from build123d import *

# Parameters (mm, degrees)
SKETCH_1_R               = 4
EXTRUDE_1_DEPTH          = 147.8
SKETCH_2_R               = 3
EXTRUDE_2_DEPTH          = 5
CUT_EXTRUDE_1_DEPTH      = 153.904676187
CUT_EXTRUDE_1_DEPTH_BACK = 153.904676187
SKETCH_3_R               = 1.65


with BuildPart() as part:
    # ｽｹｯﾁ1 → ﾎﾞｽ - 押し出し1 (new body)
    with BuildSketch(Plane.XY):
        Circle(SKETCH_1_R)
    extrude(amount=EXTRUDE_1_DEPTH)

    # ｽｹｯﾁ2 → ﾎﾞｽ - 押し出し2 (add)
    with BuildSketch(Plane.XY.offset(147.8)):
        Circle(SKETCH_2_R)
    extrude_2 = extrude(amount=EXTRUDE_2_DEPTH)

    # ﾐﾗｰ1: ﾎﾞｽ - 押し出し2 across plane
    add(extrude_2.mirror(Plane.XY.offset(73.9)))

    # ｽｹｯﾁ3 → ｶｯﾄ - 押し出し1 (cut, two sides: drawn at the far end of the back side and taken through both)
    with BuildSketch(Plane(origin=(0, 0, 0), x_dir=(1, 0, 0), z_dir=(0, 1, 0)).offset(-CUT_EXTRUDE_1_DEPTH_BACK)):
        with Locations(Location((0, -63.9, 0), (0, 0, 270))):
            Circle(SKETCH_3_R)
        with Locations(Location((0, -83.9, 0), (0, 0, 270))):
            Circle(SKETCH_3_R)
    extrude(amount=CUT_EXTRUDE_1_DEPTH + CUT_EXTRUDE_1_DEPTH_BACK, mode=Mode.SUBTRACT)


solid = part.part
Here's how the part is built. I have some questions about the finished solid (model axes, mm). A direction names the side the tool comes from. Round coordinates to 2 decimals unless told otherwise and drop trailing zeros. Order: outer loops, then holes, each group sorted by start corner. A loop starts at its lowest first (then second) coordinate and runs counter-clockwise, first axis right, second up. Notation, with made-up numbers: M -21.5,-34 L 11.5,-34 A13 ccw 11.5,-15 Z; hole C 10,76.5 d10. An arc over 180 degrees is marked long. Return JSON: item names as keys, results as strings. Group by question number.
1. On a 3-axis mill with a long thin cutter (end or side, diameter ignored), from which of +Z, -Z, +X, -X, +Y, -Y can I reach the whole of each face in a straight line? I mean faces 1 (the face through (1, 3, 0)), 2 (the face through (0, 0, -5)), 3 (the face through (-3, 0, 150)). Say none if no direction works.
2. Please list where these lines run through material, in increasing order: probe 1 along Z at (x, y) = (0, -1); probe 2 along Z at (x, y) = (0.75, 3); probe 3 along Z at (x, y) = (2, -3).
3. If we mould it in two halves opening along Z, with no side actions, what happens to faces 4 (the face through (0.496, -0.056, 65.474)), 5 (the face through (1, 3, 147.8)), 6 (the face through (-3, 0, -2))? For each: pulls with the +Z half, pulls with the -Z half, needs draft (parallel to the pull), parting line crosses it, or undercut.
4. If we section it at B-B on z = 106.5: List the corners of the cut face in (x, y) for me, then the cut area to 3 significant figures.
5. I'm going to push flat-ended pins straight in: pin 1 Ø4 at (x, z) = (1.5, 90.5) entering from -Y; pin 2 Ø3 at (y, z) = (3, 58) entering from -X; pin 3 Ø2 at (y, z) = (-1.5, 19) entering from +X. Where does each tip first touch, or does it pass through?
6. If we section it at C-C on z = 83.9: List the corners of the cut face in (x, y) for me, then the cut area to 3 significant figures.
7. If we section it at A-A on y = 0: List the corners of the cut face in (x, z) for me, then the cut area to 3 significant figures.
Reply:
{
 "1": {"face 1": "-Z", "face 2": "-Z, +X, -X, +Y, -Y", "face 3": "+Z"},
 "2": {"probe 1": "-5 to 62.25, 65.55 to 82.25, 85.55 to 152.8", "probe 2": "0 to 62.43, 65.37 to 82.43, 85.37 to 147.8", "probe 3": "0 to 147.8"},
 "3": {"face 4": "undercut", "face 5": "pulls with the +Z half", "face 6": "needs draft"},
 "4": {"outline": "C 0,0 d8", "area": "50.3 mm^2"},
 "5": {"pin 1": "y = -4", "pin 2": "x = -3.71", "pin 3": "x = 3.97"},
 "6": {"outline": "M -1.65,-3.64 L -1.65,3.64 A4 ccw Z; M 1.65,-3.64 A4 ccw 1.65,3.64 Z", "area": "24.6 mm^2"},
 "7": {"outline": "M -4,0 L -3,0 L -3,-5 L 3,-5 L 3,0 L 4,0 L 4,147.8 L 3,147.8 L 3,152.8 L -3,152.8 L -3,147.8 L -4,147.8 Z; hole C 0,63.9 d3.3; hole C 0,83.9 d3.3", "area": "1,230 mm^2"}
}
